The figure shows three views and two pictorial views of one solid part (mm, origin at its lowest corner). Answer the questions. Coordinates: 2 decimals unless noted, no trailing zeros. Write each loop counter-clockwise with the first axis right and the second up, starting at its lowest first coordinate (ties: lowest second). Pieces come first, ordered by that corner, then holes.
Item 1: Section D-D (x = 38.1) is taken. Give the vertices of the cut face in (y, z) (3 decimals), then the cut area to 3 significant figures.
Item 2: Section A-A (x = 63.5) is taken. Give the vertices of the cut face in (y, z) (3 decimals), then the cut area to 3 significant figures.
Item 3: Section C-C (y = 1.8) is taken. Give the vertices of the cut face in (x, z) (3 decimals), then the cut area to 3 significant figures.
Item 4: Section B-B (z = 21.59) is taken. Give the vertices of the cut face in (x, y) (3 decimals), then the cut area to 3 significant figures.
Item 5: Straight lines are drawn through the part: probe 1 along X at (y, z) = (1.1, 21.59) (3 decimals); probe 2 along X at (y, z) = (1.4, 25.4); probe 3 along Z at (x, y) = (61, 2.15). For each, find the intervals that lie inside material, in ascending order.
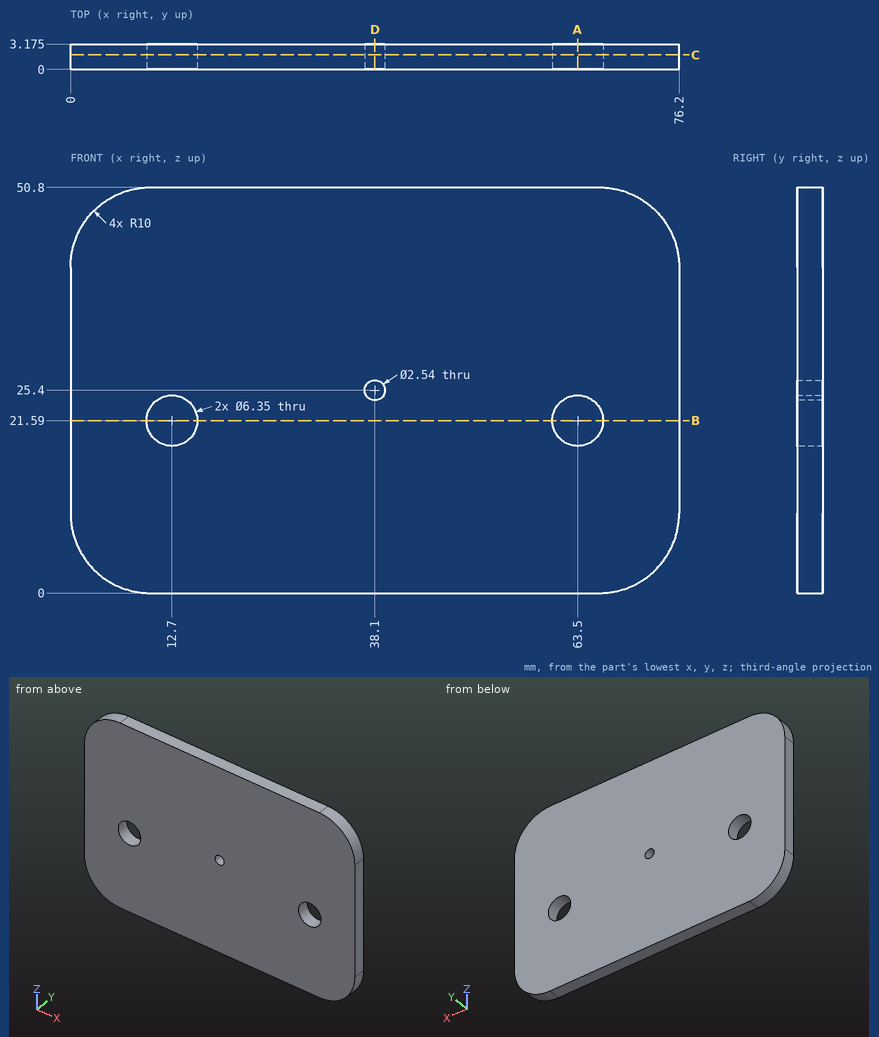
Established:
1. outline: (0, 0) - (3.175, 0) - (3.175, 24.13) - (0, 24.13) - close; (0, 26.67) - (3.175, 26.67) - (3.175, 50.8) - (0, 50.8) - close
1. area: 153 mm2
2. outline: (0, 0) - (3.175, 0) - (3.175, 18.415) - (0, 18.415) - close; (0, 24.765) - (3.175, 24.765) - (3.175, 50.8) - (0, 50.8) - close
2. area: 141 mm2
3. outline: (0, 10) arc R10 ccw to (10, 0) - (66.2, 0) arc R10 ccw to (76.2, 10) - (76.2, 40.8) arc R10 ccw to (66.2, 50.8) - (10, 50.8) arc R10 ccw to (0, 40.8) - close; hole circle Ø6.35 at (12.7, 21.59); hole circle Ø2.54 at (38.1, 25.4); hole circle Ø6.35 at (63.5, 21.59)
3. area: 3,720 mm2
4. outline: (0, 0) - (9.525, 0) - (9.525, 3.175) - (0, 3.175) - close; (15.875, 0) - (60.325, 0) - (60.325, 3.175) - (15.875, 3.175) - close; (66.675, 0) - (76.2, 0) - (76.2, 3.175) - (66.675, 3.175) - close
4. area: 202 mm2
5. probe 1: x = 0 to 9.525, 15.875 to 60.325, 66.675 to 76.2
5. probe 2: x = 0 to 36.83, 39.37 to 76.2
5. probe 3: z = 0 to 19.63, 23.55 to 50.8
